Input: part model. Units: mm. Frame: model coordinates. Face numbers are marked on the shaded views. Coordinates: 2 decimals unless noted, no trailing zeros. Order: outer loops, then holes, each group sorted by start corner. A loop starts at its lowest first (then second) coordinate and runs counter-clockwise, first axis right, second up. Notation, with made-up numbers: (42, -6) -> (55, -6) arc R24 cw to (55, 20) -> close; hole circle Ø11 at (3.25, 70). An arc over 180 degrees is marked (long way). Write each question's results on one line, items separated by ' | '.
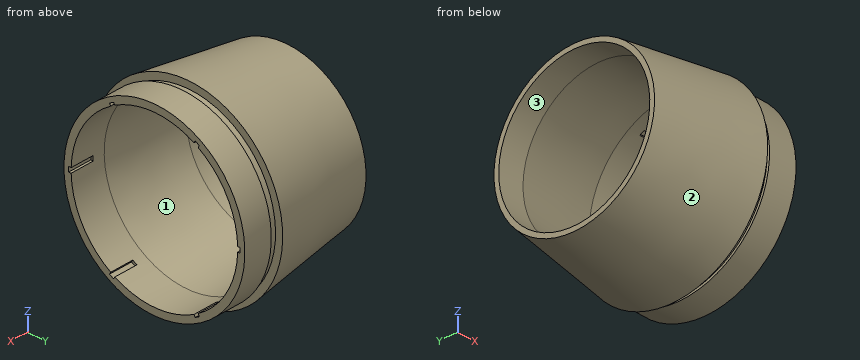
```python
from build123d import *

# Parameters (mm, degrees)
IZIM3_W                 = 10
IZIM3_H                 = 2
KES_EKSTR_ZYON1_DEPTH   = 36
DAIRESEL_KAPLAMA1_COUNT = 6


with BuildPart() as part:
    # izim1 → D_nd_r2 (revolve)
    with BuildSketch(Plane.XY, mode=Mode.PRIVATE) as d_nd_r2_sk:
        Polygon((-44.562063093, 33.737210457), (-44.562063093, 31.737210457), (-33.555064496, 31.737210457), (0, 35), (15, 35), (15, 38), (3, 38), (3, 37), (0, 37), (0, 40), align=None)
    revolve(d_nd_r2_sk.sketch.rotate(Axis((-44.316348886, 0, 0), (1, 0, 0)), 90), axis=Axis((-44.316348886, 0, 0), (1, 0, 0)))

    # izim3 → Kes-Ekstr_zyon1 (cut)
    with BuildSketch(Plane(origin=(0, 0, 0), x_dir=(1, 0, 0), z_dir=(0, 1, 0))):
        with Locations((10, 0)):
            Rectangle(IZIM3_W, IZIM3_H)
    kes_ekstr_zyon1 = extrude(amount=-KES_EKSTR_ZYON1_DEPTH, mode=Mode.SUBTRACT)

    # Dairesel Kaplama1: Kes-Ekstr_zyon1 ×6 about axis
    dairesel_kaplama1_axis = Axis((0, 0, 0), (1, 0, 0))
    for i in range(1, DAIRESEL_KAPLAMA1_COUNT):
        add(kes_ekstr_zyon1.rotate(dairesel_kaplama1_axis, i * 360 / DAIRESEL_KAPLAMA1_COUNT), mode=Mode.SUBTRACT)


solid = part.part
```
(1) Cut plane C-C, the plane x = -19. Return loops of the section in (y, z) (1 decimal).
Return value:
outline: circle Ø74.7 at (0, 0); hole circle Ø66.3 at (0, 0)
(2) Cut plane B-B, the plane x = 11. Return loops of the section in (y, z), plus the area to 3 significant figures.
Return value:
outline: circle Ø76 at (0, 0); hole (-36, -1) -> (-34.99, -1) arc R35 ccw to (-18.36, -29.8) -> (-18.87, -30.68) -> (-17.13, -31.68) -> (-16.63, -30.8) arc R35 ccw to (16.63, -30.8) -> (17.13, -31.68) -> (18.87, -30.68) -> (18.36, -29.8) arc R35 ccw to (34.99, -1) -> (36, -1) -> (36, 1) -> (34.99, 1) arc R35 ccw to (18.36, 29.8) -> (18.87, 30.68) -> (17.13, 31.68) -> (16.63, 30.8) arc R35 ccw to (-16.63, 30.8) -> (-17.13, 31.68) -> (-18.87, 30.68) -> (-18.36, 29.8) arc R35 ccw to (-34.99, 1) -> (-36, 1) -> close | area: 676 mm2
(3) Pin query (flat end, axial travel): P1, Ø0.6, axis at x = 8, z = 0.5, coming from the -Y side; P2, Ø1.5, axis at x = -26, y = -22.5, coming from the -Z side; P3, Ø8, axis at x = 4.5, z = 15.5, coming from the -Y side; P4, Ø23, axis at y = 0.5, z = -15, coming from the -X side. Return the tip coordinate at first contact, or that it passes through.
Return value:
P1: y = -38 | P2: z = -29.14 | P3: y = -36.22 | P4: through
(4) Mould query, pull axis Y, two halves, no side actions, for the marked faces 1, 2 and 3. Classes: +Y half, -Y half, draft (parallel to the pull), parting line (faces both ways), or undercut.
Return value:
face 1: undercut | face 2: parting line | face 3: undercut
(5) Line query: line 1 along Y through (x, z) = (12, 17); line 2 along Y through (x, z) = (-34, -26); line 3 along Z through (x, y) = (-11, -25.5). Output: solid intervals per line, ascending. Write a range as from..to.
Return value:
line 1: -33.99..-30.59, 30.59..33.99 | line 2: -23.76..-18.2, 18.2..23.76 | line 3: -28.78..-22.38, 22.38..28.78
(6) Cut plane A-A, the plane y = 0. Return loops of the section in (x, z), plus the area to 3 significant figures.
Return value:
outline: (-44.56, -33.74) -> (0, -40) -> (0, -37) -> (3, -37) -> (3, -38) -> (15, -38) -> (15, -35) -> (0, -35) -> (-33.56, -31.74) -> (-44.56, -31.74) -> close; (-44.56, 31.74) -> (-33.56, 31.74) -> (0, 35) -> (15, 35) -> (15, 38) -> (3, 38) -> (3, 37) -> (0, 37) -> (0, 40) -> (-44.56, 33.74) -> close | area: 432 mm2
(7) Cut plane D-D, the plane x = -10. Return loops of the section in (y, z), plus the area to 3 significant figures.
Return value:
outline: circle Ø77.19 at (0, 0); hole circle Ø68.06 at (0, 0) | area: 1,040 mm2
